Autodesk Inventor part; units mm, degrees
ref_plane "bolt_to_nut_XY" through (25, 0, 0) normal (1, 0, 0) x (0, 0, -1)
ref_plane "bolt_to_nut_YZ" through (25, 0, 0) normal (0, 0, -1) x (0, 1, 0)
ref_plane "bolt_to_nut_ZX" through (25, 0, 0) normal (0, 1, 0) x (1, 0, 0)
sketch "Sketch_2" plane through (0, 0, 0) normal (0, 0, 1) x (1, 0, 0)
  line L0 (25, 0) -> (-3, 0)
  line L1 (-3, 0) -> (-3, 2.45)
  line L2 (-3, 2.45) -> (-2.7, 2.75)
  line L3 (-2.7, 2.75) -> (0, 2.75)
  line L4 (0, 2.75) -> (0, 1.5)
  line L5 (0, 1.5) -> (24.6935, 1.5)
  line L6 (24.6935, 1.5) -> (25, 1.1935)
  line L7 (25, 1.1935) -> (25, 0)
  line L8 (25, 0) -> (-3, 0)
revolve "Revolution1" add sketch "Sketch_2" angle 360 about axis through (25, 0, 0) along (1, 0, 0)
thread "Thread1"
sketch "Sketch2" plane through (-3, 0, 0) normal (-1, 0, 0) x (0, 0, 1)
  point P0 (0, 0)
hole "Hole1" at (-3, 0, 0) direction (1, 0, 0) diameter 2.5 depth 1.5 tip angle 150
sketch "Sketch_3" plane through (-3, 0, 0) normal (1, 0, 0) x (0, 0, -1)
  line L0 (-1.25, -0.7217) -> (0, -1.4434)
  line L1 (0, -1.4434) -> (1.25, -0.7217)
  line L2 (1.25, -0.7217) -> (1.25, 0.7217)
  line L3 (1.25, 0.7217) -> (0, 1.4434)
  line L4 (0, 1.4434) -> (-1.25, 0.7217)
  line L5 (-1.25, 0.7217) -> (-1.25, -0.7217)
extrude "Extrusion1" cut sketch "Sketch_3" along normal blind 1.5
ref_plane "bolt_to_nut_XY" through (25, 0, 0) normal (1, 0, 0) x (0, 0, -1)
ref_plane "bolt_to_nut_YZ" through (25, 0, 0) normal (0, 0, -1) x (0, 1, 0)
ref_plane "bolt_to_nut_ZX" through (25, 0, 0) normal (0, 1, 0) x (1, 0, 0)
ref_plane "screw1_XY" through (0, 0, 0) normal (1, 0, 0) x (0, 0, -1)
ref_plane "screw1_YZ" through (0, 0, 0) normal (0, 0, -1) x (0, 1, 0)
ref_plane "screw1_ZX" through (0, 0, 0) normal (0, 1, 0) x (1, 0, 0)
properties part number "CB3-25" material "鋼、炭素鋼"
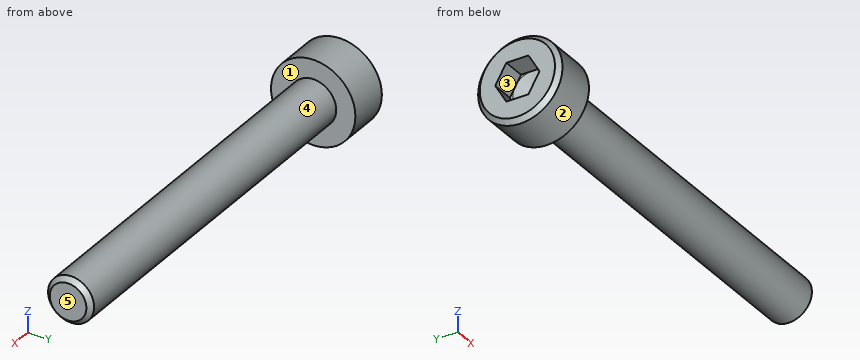
Source: CAD feature listing. Evaluate the final solid. Frame: model axes, mm. Face numbers are marked on the shaded views. A direction names the side the tool comes from. Give positions to 0.01 mm unless a question says otherwise; leave off trailing zeros. Write each loop counter-clockwise with the first axis right and the second up, starting at its lowest first coordinate (ties: lowest second). Pieces come first, ordered by that corner, then holes. Notation, with made-up numbers: M -15.5,51 L 32.5,51 A14 ccw 32.5,61 Z; hole C 23.25,-24 d4. An arc over 180 degrees is marked long. Return JSON: item names as keys, results as strings. Group by question number.
1) Cut plane A-A, the plane x = 5.5. Output: boundary loops of the cut face in (y, z), plus the area to 3 significant figures.
2) Pull-direction query (Y, two-part tool) for the marked faces 3, 4 and 5; classes: pulls with the +Y half, pulls with the -Y half, needs draft (parallel to the pull), parting line crosses it, or undercut.
3) Material intervals for line 1 along Z through (x, y) = (14.75, -0.9); line 2 along X through (y, z) = (1.6, 1.75); line 3 along Y through (x, z) = (19.25, -0.1), sorted ascending. Write a range as [from, to].
4) Set-up query: the marked faces 1 and 2. Return all of +Z, -Z, +X, -X, +Y, -Y with unobstructed straight access to the full face (end or side cutting, diameter ignored); none if empty.
5) Pin query (flat end, axial travel): P1, Ø2, axis at x = 3, y = -0.5, coming from the -Z side; P2, Ø1.5, axis at y = -0.5, z = 2, coming from the +X side; P3, Ø1.2, axis at y = -0.5, z = 0, coming from the -X side. Return the tip coordinate at first contact, or that it passes through.
Recorded:
{
 "1": {"outline": "C 0,0 d3", "area": "7.07 mm²"},
 "2": {"face 3": "undercut", "face 4": "parting line crosses it", "face 5": "needs draft"},
 "3": {"line 1": "z = [-1.2, 1.2]", "line 2": "x = [-3, 0]", "line 3": "y = [-1.5, 1.5]"},
 "4": {"face 1": "+X", "face 2": "+X, -X"},
 "5": {"P1": "stops at z = -1.5", "P2": "stops at x = 24.88", "P3": "stops at x = -1.46"}
}
